Check sheet for the modelled part. Datum: model origin and axes. Units: mm. Face numbers are marked on the shaded views. A direction names the side the tool comes from. Round coordinates to 2 decimals unless told otherwise and drop trailing zeros. Order: outer loops, then holes, each group sorted by start corner. A loop starts at its lowest first (then second) coordinate and runs counter-clockwise, first axis right, second up. Notation, with made-up numbers: (18.25, -8) -> (28.25, -8) arc R3 ccw to (28.25, -3) -> close; hole circle Ø9 at (7, -21.75). An arc over 180 degrees is marked (long way). Answer in a Markdown table with one row per item.
from build123d import *

# Parameters (mm, degrees)
EXTRU_MINCE1_DEPTH      = 8
ENL_V_MAT_EXTRU_1_REACH = 45.174
ESQUISSE2_R             = 1.6
ENL_V_MAT_EXTRU_2_DEPTH = 5.5
ENL_V_MAT_EXTRU_3_REACH = 45.174
ESQUISSE4_R             = 1.6
ENL_V_MAT_EXTRU_4_DEPTH = 5.5
CONG_1_R                = 1


with BuildPart() as part:
    # Esquisse1 → Extru.-Mince1 (new body)
    with BuildSketch(Plane(origin=(0, 0, 0), x_dir=(1, 0, 0), z_dir=(0, 1, 0))):
        with BuildLine():
            Line((30, 0), (9, 0))
            ThreePointArc((9, 0), (2.636038969, -2.636038969), (0, -9))
            Line((0, -9), (0, -30))
            Line((0, -30), (8, -30))
            Line((8, -30), (8, -9))
            ThreePointArc((8, -9), (8.292893219, -8.292893219), (9, -8))
            Line((9, -8), (30, -8))
            Line((30, -8), (30, 0))
        make_face()
    extrude(amount=EXTRU_MINCE1_DEPTH)

    # Esquisse2 → Enlèv. mat.-Extru.1 (cut, up to next)
    with BuildSketch(Plane.XZ, mode=Mode.PRIVATE) as enl_v_mat_extru_1_sk1:
        with Locations(Location((18, 4, 0), (0, 0, 270))):
            Circle(ESQUISSE2_R)
    enl_v_mat_extru_1_tool1 = extrude(enl_v_mat_extru_1_sk1.sketch, amount=-ENL_V_MAT_EXTRU_1_REACH, mode=Mode.PRIVATE) & part.part
    # Esquisse2 → Enlèv. mat.-Extru.1 (cut, up to next)
    with BuildSketch(Plane.XZ, mode=Mode.PRIVATE) as enl_v_mat_extru_1_sk2:
        with Locations(Location((4, 18, 0), (0, 0, 270))):
            Circle(ESQUISSE2_R)
    enl_v_mat_extru_1_tool2 = extrude(enl_v_mat_extru_1_sk2.sketch, amount=-ENL_V_MAT_EXTRU_1_REACH, mode=Mode.PRIVATE) & part.part
    add(enl_v_mat_extru_1_tool1.solids().sort_by_distance((18, 0, 4))[0], mode=Mode.SUBTRACT)
    add(enl_v_mat_extru_1_tool2.solids().sort_by_distance((4, 0, 18))[0], mode=Mode.SUBTRACT)

    # Esquisse3 → Enlèv. mat.-Extru.2 (cut)
    with BuildSketch(Plane(origin=(0, 8, 0), x_dir=(1, 0, 0), z_dir=(0, 1, 0))):
        Polygon((5.616580754, -20.8), (7.233161507, -18), (5.616580754, -15.2), (2.383419246, -15.2), (0.766838493, -18), (2.383419246, -20.8), align=None)
        Polygon((19.616580754, -6.8), (21.233161507, -4), (19.616580754, -1.2), (16.383419246, -1.2), (14.766838493, -4), (16.383419246, -6.8), align=None)
    extrude(amount=-ENL_V_MAT_EXTRU_2_DEPTH, mode=Mode.SUBTRACT)

    # Esquisse4 → Enlèv. mat.-Extru.3 (cut, up to next)
    with BuildSketch(Plane(origin=(0, 0, 0), x_dir=(-1, 0, 0), z_dir=(0, 0, -1)), mode=Mode.PRIVATE) as enl_v_mat_extru_3_sk1:
        with Locations((-26, 4)):
            Circle(ESQUISSE4_R)
    enl_v_mat_extru_3_tool1 = extrude(enl_v_mat_extru_3_sk1.sketch, amount=-ENL_V_MAT_EXTRU_3_REACH, mode=Mode.PRIVATE) & part.part
    enl_v_mat_extru_3 = enl_v_mat_extru_3_tool1.solids().sort_by_distance((26, 4, 0))[0]
    add(enl_v_mat_extru_3, mode=Mode.SUBTRACT)

    # Esquisse5 → Enlèv. mat.-Extru.4 (cut)
    with BuildSketch(Plane.XY.offset(8)):
        Polygon((27.616580754, 1.2), (29.233161507, 4), (27.616580754, 6.8), (24.383419246, 6.8), (22.766838493, 4), (24.383419246, 1.2), align=None)
    enl_v_mat_extru_4 = extrude(amount=-ENL_V_MAT_EXTRU_4_DEPTH, mode=Mode.SUBTRACT)

    # Symétrie1: Enlèv. mat.-Extru.3, Enlèv. mat.-Extru.4 across plane
    add(enl_v_mat_extru_3.mirror(Plane(origin=(0, 0, 0), x_dir=(0.7071067811865476, 0, 0.7071067811865475), z_dir=(0.7071067811865475, 0, -0.7071067811865476))), mode=Mode.SUBTRACT)
    add(enl_v_mat_extru_4.mirror(Plane(origin=(0, 0, 0), x_dir=(0.7071067811865476, 0, 0.7071067811865475), z_dir=(0.7071067811865475, 0, -0.7071067811865476))), mode=Mode.SUBTRACT)

    # Congé1
    # the kernel refuses this fillet: 1 mm, written as the material it takes off along each edge
    with BuildSketch(Plane(origin=(7, 7, 29), x_dir=(0, 1, 0), z_dir=(1, 0, 0))) as cong_1_piece_1_section:
        Polygon((0, 0), (CONG_1_R, 0), (CONG_1_R, CONG_1_R), (0, CONG_1_R), align=None)
    cong_1_piece_1 = extrude(amount=CONG_1_R, mode=Mode.PRIVATE)
    cong_1_piece_1 = cong_1_piece_1 - Plane(origin=(7, 7, 29), x_dir=(0, -0.7071067811865475, -0.7071067811865475), z_dir=(1, 0, 0)) * Sphere(CONG_1_R, mode=Mode.PRIVATE)
    add(cong_1_piece_1, mode=Mode.SUBTRACT)
    with BuildSketch(Plane(origin=(29, 7, 7), x_dir=(0, 1, 0), z_dir=(0, 0, 1))) as cong_1_piece_2_section:
        Polygon((0, 0), (CONG_1_R, 0), (CONG_1_R, -CONG_1_R), (0, -CONG_1_R), align=None)
    cong_1_piece_2 = extrude(amount=CONG_1_R, mode=Mode.PRIVATE)
    cong_1_piece_2 = cong_1_piece_2 - Plane(origin=(29, 7, 7), x_dir=(-0.7071067811865475, -0.7071067811865475, 0), z_dir=(0, 0, 1)) * Sphere(CONG_1_R, mode=Mode.PRIVATE)
    add(cong_1_piece_2, mode=Mode.SUBTRACT)
    with BuildSketch(Plane(origin=(8, 8, 29), x_dir=(-1, 0, 0), z_dir=(0, 0, -1))) as cong_1_piece_3:
        with BuildLine():
            CenterArc((CONG_1_R, -CONG_1_R), CONG_1_R, 90, 90)
            Line((0, -CONG_1_R), (0, 0))
            Line((0, 0), (CONG_1_R, 0))
        make_face()
    extrude(amount=20, mode=Mode.SUBTRACT)
    with BuildSketch(Plane(origin=(30, -2.5, 8), x_dir=(-1, 0, 0), z_dir=(0, 1, 0)), Plane(origin=(30, 8, 7), x_dir=(-1, 0, 0), z_dir=(0, 0, -1)), Plane(origin=(-2.5, 8, 30), x_dir=(0, 0, -1), z_dir=(1, 0, 0))) as cong_1_piece_4:
        with BuildLine():
            CenterArc((CONG_1_R, -CONG_1_R), CONG_1_R, 90, 90)
            Line((0, -CONG_1_R), (0, 0))
            Line((0, 0), (CONG_1_R, 0))
        make_face()
    extrude(amount=9.5, mode=Mode.SUBTRACT)
    with BuildSketch(Plane(origin=(8, -2.5, 30), x_dir=(0, 0, -1), z_dir=(0, 1, 0))) as cong_1_piece_5:
        with BuildLine():
            CenterArc((CONG_1_R, CONG_1_R), CONG_1_R, 180, 90)
            Line((0, CONG_1_R), (0, 0))
            Line((0, 0), (CONG_1_R, 0))
        make_face()
    extrude(amount=9.5, mode=Mode.SUBTRACT)
    with BuildSketch(Plane(origin=(9, 8, 9), x_dir=(-1, 0, 0), z_dir=(0, 0, 1))) as cong_1_piece_6:
        with BuildLine():
            CenterArc((1 + CONG_1_R, CONG_1_R), CONG_1_R, 180, 90)
            Line((1 + CONG_1_R, 0), (1, 0))
            Line((1, 0), (1, CONG_1_R))
        make_face()
    revolve(axis=Axis((9, 8, 9), (0, -1, 0)), revolution_arc=90, mode=Mode.SUBTRACT)
    with BuildSketch(Plane(origin=(9, 8, 8), x_dir=(0, -1, 0), z_dir=(1, 0, 0))) as cong_1_piece_7:
        with BuildLine():
            CenterArc((CONG_1_R, CONG_1_R), CONG_1_R, 180, 90)
            Line((0, CONG_1_R), (0, 0))
            Line((0, 0), (CONG_1_R, 0))
        make_face()
    extrude(amount=20, mode=Mode.SUBTRACT)


solid = part.part
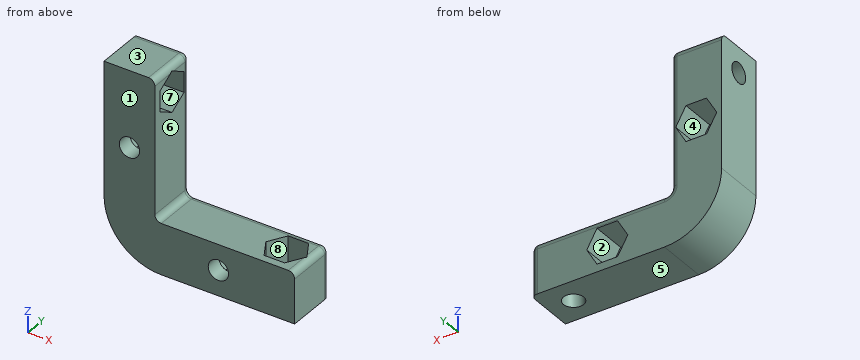
Item 1: Cross-section at C-C (x = 4). Record the boundary of the cut face in (y, z).
Result sheet:
| item | result |
|---|---|
| outline | (0, 1.52) -> (8, 1.52) -> (8, 15.2) -> (2.5, 15.2) -> (2.5, 16.4) -> (0, 16.4) -> close; (0, 19.6) -> (2.5, 19.6) -> (2.5, 20.8) -> (8, 20.8) -> (8, 29) arc R1 ccw to (7, 30) -> (0, 30) -> close; hole (1.2, 24.38) -> (4, 22.77) -> (6.8, 24.38) -> (6.8, 27.62) -> (4, 29.23) -> (1.2, 27.62) -> close |
Item 2: Scan lines: line 1 (X direction, y = 1.95, z = 4); line 2 (Z direction, x = 1.6, y = 4); line 3 (X direction, y = 1.35, z = 4). Record each from-to range of solid material in increasing order. Write a range as [from, to].
Result sheet:
| item | result |
|---|---|
| line 1 | x = [1.52, 16.4], [19.6, 23.95], [28.05, 30] |
| line 2 | z = [3.88, 16.56], [19.44, 24.4], [27.6, 30] |
| line 3 | x = [1.52, 16.4], [19.6, 24.3], [27.7, 30] |
Item 3: Depth check by flat-ended pin: P1, Ø1.7, axis at x = 17, z = 3, coming from the +Y side; P2, Ø1, axis at x = 18, y = 5, coming from the +Z side; P3, Ø2, axis at y = 4, z = 23, coming from the +X side; P4, Ø3, axis at x = 18, z = 4, coming from the -Y side. Enter the tip coordinate at first touch or a pass-through.
Result sheet:
| item | result |
|---|---|
| P1 | stops at y = 2.5 |
| P2 | stops at z = 8 |
| P3 | stops at x = 8 |
| P4 | passes through |
Item 4: Cross-section at D-D (z = 22). Record the boundary of the cut face in (x, y).
Result sheet:
| item | result |
|---|---|
| outline | (0, 0) -> (8, 0) -> (8, 7) arc R1 ccw to (7, 8) -> (0, 8) -> close |
Item 5: Set-up check for the marked faces 4, 5, 6, 7 and 8: record each of +Z, -Z, +X, -X, +Y, -Y from which the full face is reachable in a straight line by a thin tool's end or side.
Result sheet:
| item | result |
|---|---|
| face 4 | +Y |
| face 5 | -Z, +X, -X, +Y, -Y |
| face 6 | +Z, +X, +Y, -Y |
| face 7 | +X |
| face 8 | +Z |
Item 6: Cross-section at A-A (z = 26). Record the boundary of the cut face in (x, y), and give its area (3 significant figures).
Result sheet:
| item | result |
|---|---|
| outline | (0, 0) -> (8, 0) -> (8, 1.2) -> (2.5, 1.2) -> (2.5, 2.4) -> (0, 2.4) -> close; (0, 5.6) -> (2.5, 5.6) -> (2.5, 6.8) -> (8, 6.8) -> (8, 7) arc R1 ccw to (7, 8) -> (0, 8) -> close |
| area | 25.0 mm^2 |
Item 7: Cross-section at B-B (x = 26). Record the boundary of the cut face in (y, z).
Result sheet:
| item | result |
|---|---|
| outline | (0, 0) -> (2.4, 0) -> (2.4, 2.5) -> (1.2, 2.5) -> (1.2, 8) -> (0, 8) -> close; (5.6, 0) -> (8, 0) -> (8, 7) arc R1 ccw to (7, 8) -> (6.8, 8) -> (6.8, 2.5) -> (5.6, 2.5) -> close |
Item 8: Mould release check, pull along Z, two halves, no side actions. Record for the marked faces 1, 2 and 3: pulls with the +Z half, pulls with the -Z half, needs draft (parallel to the pull), parting line crosses it, or undercut.
Result sheet:
| item | result |
|---|---|
| face 1 | needs draft |
| face 2 | undercut |
| face 3 | pulls with the +Z half |
